```python
from build123d import *

# Parameters (mm, degrees)
F0_W     = 55
F0_H     = 32
F1_DEPTH = 40
F2_W     = 30
F2_H     = 18
F3_DEPTH = 20
F4_W     = 30
F4_H     = 18
F5_DEPTH = 20
F6_R     = 5
F7_DEPTH = 20.001
F8_SIZE  = 5
F9_R     = 3


with BuildPart() as f1:
    # F0 (on Front) → F1 (new body)
    with BuildSketch(Plane.XZ):
        with Locations((27.5, -16)):
            Rectangle(F0_W, F0_H)
    extrude(amount=F1_DEPTH)

    # F2 (on Front) → F3 (cut)
    with BuildSketch(Plane.XZ):
        with Locations((35.8558194712, -20.2440911922)):
            Rectangle(F2_W, F2_H)
    extrude(amount=-F3_DEPTH, mode=Mode.SUBTRACT)

    # F4 (on face) → F5 (cut)
    with BuildSketch(Plane.XZ.offset(40)):
        with Locations((40, -23)):
            Rectangle(F4_W, F4_H)
    extrude(amount=-F5_DEPTH, mode=Mode.SUBTRACT)

    # F6 (on face) → F7 (cut, through all)
    with BuildSketch(Plane.XZ.offset(20)):
        with Locations((35, -19)):
            Circle(F6_R)
    extrude(amount=-F7_DEPTH, mode=Mode.SUBTRACT)

    # F8
    f8_edges = [f1.edges().sort_by_distance(p)[0] for p in [
        (12.5, -40, -32),
        (25, -40, -23),
        (40, -40, -14),
        (55, -40, -7),
        (0, -40, -16),
        (27.5, -40, 0),
    ]]
    chamfer(f8_edges, length=F8_SIZE)

    # F9
    f9_edges = [f1.edges().sort_by_distance(p)[0] for p in [
        (0, -35, -16),
        (12.5, -35, -32),
        (25, -35, -23),
        (40, -35, -14),
        (55, -35, -7),
        (27.5, -35, 0),
    ]]
    fillet(f9_edges, radius=F9_R)


solid = f1.part
```
Source: CAD feature listing. Evaluate the final solid. Frame: model axes, mm. A direction names the side the tool comes from. Coordinates: 2 decimals unless noted, no trailing zeros. Loops run counter-clockwise (first coordinate to the right, second up) from the corner with the lowest first, then second, coordinate; pieces in that order, holes last. Notation, with made-up numbers: M 19.5,82 L 67.5,82 A35 cw 67.5,118 Z; hole C 69,71.25 d5. An arc over 180 degrees is marked long. Use a Markdown table: item, result. Add a question column.
Q1. Access query for faces 1 (the cylindrical face through (54.78, -34.89, -6.9)), 2 (the cylindrical face through (39.78, -34.89, -13.78)). Directions: +Z, -Z, +X, -X, +Y, -Y. A direction counts if a zero-diameter tool reaches every point of the face in a straight line with its end or side. Return the directions, or none.
Q2. Material intervals for L1, parallel to X at y = -15.5, z = -19; L2, parallel to Z at x = 35, y = -11.5; L3, parallel to X at y = -5, z = -15.5, sorted ascending.
Q3. Section query C-C, the plane y = -12.5. Return loops of the section in (x, z), and give its area (3 significant figures).
Q4. Section query D-D, the plane z = -10. Return loops of the section in (x, y).
Q5. Section query A-A, the plane z = -23. Return loops of the section in (x, y), and give its area (3 significant figures).
Q6. Section query B-B, the plane x = 45. Return loops of the section in (y, z), and give its area (3 significant figures).
Q7. First-contact query: pin 1 (9 mm diameter, centred on x = 45, z = -24.5, fed in from -Y); pin 2 (7 mm diameter, centred on y = -25, z = -23, fed in from +X); pin 3 (12 mm diameter, centred on x = 41, y = -27, fed in from -Z). Flat tips, straight axial feed; report the tip coordinate or a pass-through.
Result:
| question | item | result |
|---|---|---|
| 1 | face 1 | +Z, -Z, +X, -Y |
| 1 | face 2 | -Z, +X, -Y |
| 2 | L1 | x = 0 to 30, 40 to 55 |
| 2 | L2 | z = -32 to -24, -14 to 0 |
| 2 | L3 | x = 0 to 31.43, 38.57 to 55 |
| 3 | outline | M 0,-32 L 55,-32 L 55,0 L 0,0 Z; hole C 35,-19 d10 |
| 3 | area | 1,680 mm2 |
| 4 | outline | M 0,-33.76 A3 ccw 0.88,-35.88 L 5,-40 L 20,-40 L 21,-39 L 51,-39 L 54.12,-35.88 A3 ccw 55,-33.76 L 55,0 L 0,0 Z |
| 5 | outline | M 0,-33.76 A3 ccw 0.88,-35.88 L 5,-40 L 20,-40 L 24.12,-35.88 A3 ccw 25,-33.76 L 25,-20 L 32,-20 L 32,0 L 0,0 Z; M 38,-20 L 55,-20 L 55,0 L 38,0 Z |
| 5 | area | 1,450 mm2 |
| 6 | outline | M -40,-9 L -35.88,-13.12 A3 ccw -33.76,-14 L -20,-14 L -20,-32 L 0,-32 L 0,0 L -33.76,0 A3 ccw -35.88,-0.88 L -40,-5 Z |
| 6 | area | 895 mm2 |
| 7 | pin 1 | stops at y = -20 |
| 7 | pin 2 | stops at x = 25 |
| 7 | pin 3 | stops at z = -14 |
